The figure shows three views and two pictorial views of one solid part (mm, origin at its lowest corner). Answer the questions. Coordinates: 2 decimals unless noted, no trailing zeros. Write each loop counter-clockwise with the first axis right and the second up, starting at its lowest first coordinate (ties: lowest second). Pieces come first, ordered by that corner, then holes.
Item 1: Each of these flat-tipped pins is pushed along its axis until it touches: P1, Ø5, axis at x = 106, z = 6, coming from the +Y side; P2, Ø4.5, axis at x = 189, y = 29.5, coming from the +Z side; P3, Ø4, axis at x = 128, z = 3, coming from the +Y side; P4, Ø8, axis at x = 10, y = 29.5, coming from the -Z side. Where does it stop, or does it pass through?
Item 2: Section C-C (y = 47) is taken. Give the vertices of the cut face in (x, z), then the cut area to 3 significant figures.
Item 3: Section A-A (y = 29.5) is taken. Give the vertices of the cut face in (x, z).
Item 4: Section B-B (x = 189) is taken. Give the vertices of the cut face in (y, z), then the cut area to 3 significant figures.
Item 5: Straight lines are drawn through the part: probe 1 along Y at (x, z) = (10, 10.6); probe 2 along X at (y, z) = (40.5, 1.75); probe 3 along Y at (x, z) = (44.5, 3.5). For each, find the intervals that lie inside material, in ascending order.
Item 6: Section D-D (x = 131.5) is taken. Give the vertices of the cut face in (y, z).
Item 7: Determine the mould class of the marked faces 1 and 2 for opening direction X: released by +X, released by -X, zero draft, split by the parting line, or undercut.
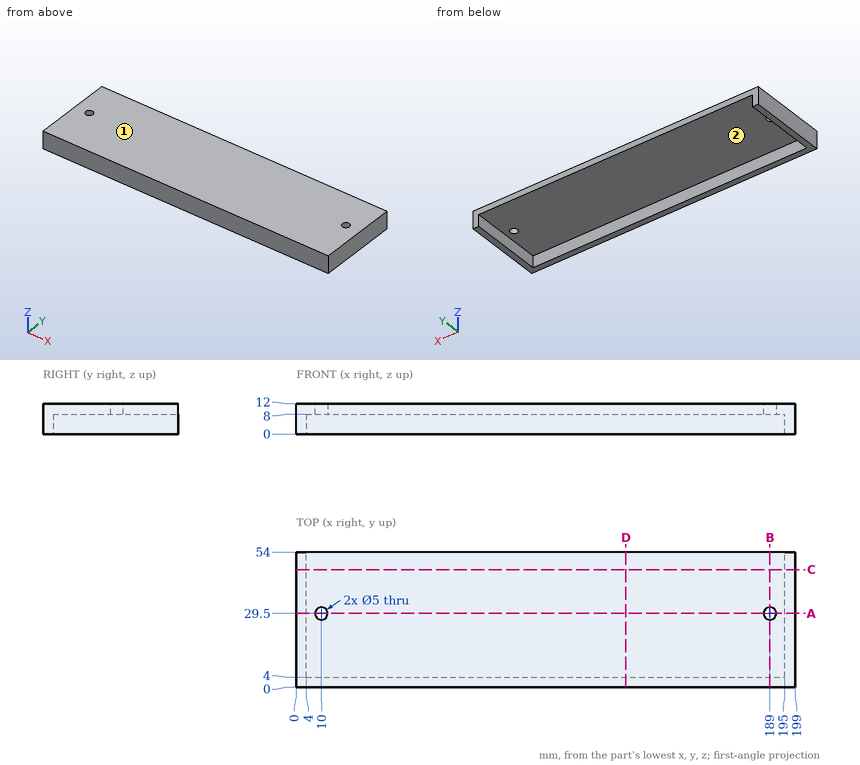
Established:
1. P1: stops at y = 54
1. P2: passes through
1. P3: stops at y = 4
1. P4: stops at z = 8
2. outline: (0, 0) - (4, 0) - (4, 8) - (195, 8) - (195, 0) - (199, 0) - (199, 12) - (0, 12) - close
2. area: 860 mm2
3. outline: (0, 0) - (4, 0) - (4, 8) - (7.5, 8) - (7.5, 12) - (0, 12) - close; (12.5, 8) - (186.5, 8) - (186.5, 12) - (12.5, 12) - close; (191.5, 8) - (195, 8) - (195, 0) - (199, 0) - (199, 12) - (191.5, 12) - close
4. outline: (0, 0) - (4, 0) - (4, 8) - (27, 8) - (27, 12) - (0, 12) - close; (32, 8) - (54, 8) - (54, 12) - (32, 12) - close
4. area: 228 mm2
5. probe 1: y = 0 to 27, 32 to 54
5. probe 2: x = 0 to 4, 195 to 199
5. probe 3: y = 0 to 4
6. outline: (0, 0) - (4, 0) - (4, 8) - (54, 8) - (54, 12) - (0, 12) - close
7. face 1: zero draft
7. face 2: undercut
